Geometry check sheet. Reference: the model listing, model coordinates, mm. A direction names the side the tool comes from. Round coordinates to 2 decimals unless told otherwise and drop trailing zeros. Write each loop counter-clockwise with the first axis right and the second up, starting at its lowest first coordinate (ties: lowest second). Pieces come first, ordered by that corner, then holes. Notation, with made-up numbers: (-33, 6) -> (9, 6) arc R21 cw to (9, 23) -> close; hole circle Ø11 at (75, -39). An arc over 180 degrees is marked (long way). Use a Markdown table: item, result.
```python
from build123d import *

# Parameters (mm, degrees)
SKETCH2_R                        = 31.5
BOSS_EXTRUDE1_DEPTH              = 12
CBORE_FOR_M6_SHCS1_D             = 6.6
CBORE_FOR_M6_SHCS1_CBORE_D       = 11
CBORE_FOR_M6_SHCS1_CBORE_DEPTH   = 6.5
SKETCH5_R                        = 3.15
CUT_EXTRUDE1_DEPTH               = 6.5
BOSS_EXTRUDE2_DEPTH              = 27
CBORE_FOR_M2_5_SHCS1_D           = 2.7
CBORE_FOR_M2_5_SHCS1_CBORE_D     = 5.5
CBORE_FOR_M2_5_SHCS1_CBORE_DEPTH = 2.5
SKETCH9_W                        = 14.384523908
SKETCH9_H                        = 27
SKETCH9_W_2                      = 10
SKETCH9_H_2                      = 6
SKETCH9_W_3                      = 11.37493753
CUT_EXTRUDE2_DEPTH               = 15


with BuildPart() as part:
    # Sketch2 → Boss-Extrude1 (new body)
    with BuildSketch(Plane.XY):
        Circle(SKETCH2_R)
    extrude(amount=BOSS_EXTRUDE1_DEPTH)

    # CBORE for M6 SHCS1 (through all)
    with Locations(Plane.XY.offset(12)):
        with Locations((0, 25), (0, -25)):
            CounterBoreHole(CBORE_FOR_M6_SHCS1_D / 2, CBORE_FOR_M6_SHCS1_CBORE_D / 2, CBORE_FOR_M6_SHCS1_CBORE_DEPTH)

    # Sketch5 → Cut-Extrude1 (cut)
    with BuildSketch(Plane(origin=(0, 0, 0), x_dir=(-1, 0, 0), z_dir=(0, 0, -1))):
        with Locations((17.67766953, 17.67766953)):
            Circle(SKETCH5_R)
    extrude(amount=-CUT_EXTRUDE1_DEPTH, mode=Mode.SUBTRACT)

    # Sketch6 → Boss-Extrude2 (add)
    with BuildSketch(Plane(origin=(0, 0, 12), x_dir=(-1, 0, 0), z_dir=(0, 0, -1))):
        with BuildLine():
            Line((-31.379730719, -2.75), (31.379730719, -2.75))
            ThreePointArc((31.379730719, -2.75), (29.665019709, -10.594177913), (26.022826518, -17.75))
            Line((26.022826518, -17.75), (-26.022826518, -17.75))
            ThreePointArc((-26.022826518, -17.75), (-29.665019709, -10.594177913), (-31.379730719, -2.75))
        make_face()
    extrude(amount=-BOSS_EXTRUDE2_DEPTH)

    # CBORE for M2.5 SHCS1 (through all)
    with Locations(Plane(origin=(0, -2.75, 0), x_dir=(1, 0, 0), z_dir=(0, 1, 0))):
        with Locations((-9.995206811, -25), (14.004793189, -37), (-9.995206811, -37), (14.004793189, -25)):
            CounterBoreHole(CBORE_FOR_M2_5_SHCS1_D / 2, CBORE_FOR_M2_5_SHCS1_CBORE_D / 2, CBORE_FOR_M2_5_SHCS1_CBORE_DEPTH)

    # Sketch9 → Cut-Extrude2 (cut)
    with BuildSketch(Plane(origin=(0, -2.75, 0), x_dir=(1, 0, 0), z_dir=(0, 1, 0))):
        with Locations((-24.187468765, -25.5)):
            Rectangle(SKETCH9_W, SKETCH9_H)
        with Locations((6.504793189, -36)):
            Rectangle(SKETCH9_W_2, SKETCH9_H_2)
        with Locations((25.692261954, -36)):
            Rectangle(SKETCH9_W_3, SKETCH9_H_2)
    extrude(amount=-CUT_EXTRUDE2_DEPTH, mode=Mode.SUBTRACT)


solid = part.part
```
(1) Section check D-D on y = -16. Record the cut outline in (x, z), plus the area to 3 significant figures.
A:
| item | result |
|---|---|
| outline | (-27.13, 0) -> (27.13, 0) -> (27.13, 33) -> (20, 33) -> (20, 39) -> (11.5, 39) -> (11.5, 33) -> (1.5, 33) -> (1.5, 39) -> (-17, 39) -> (-17, 12) -> (-27.13, 12) -> close; hole circle Ø2.7 at (-10, 25); hole circle Ø2.7 at (-10, 37); hole circle Ø2.7 at (14, 25); hole circle Ø2.7 at (14, 37) |
| area | 1,720 mm2 |
(2) Access from +Z, -Z, +X, -X, +Y, -Y to the whole of each face (thin tool, end or side, straight path). Record for faces 1 (the face through (-9.9, -3.98, 34.25)), 2 (the face through (0, 21, 5.5)), 3 (the face through (-18, 18, 6.5)).
A:
| item | result |
|---|---|
| face 1 | +Y |
| face 2 | +Z |
| face 3 | -Z |
(3) Section check C-C on y = -25. Record the cut outline in (x, z).
A:
| item | result |
|---|---|
| outline | (-19.16, 0) -> (-3.3, 0) -> (-3.3, 5.5) -> (-5.5, 5.5) -> (-5.5, 12) -> (-19.16, 12) -> close; (3.3, 0) -> (19.16, 0) -> (19.16, 12) -> (5.5, 12) -> (5.5, 5.5) -> (3.3, 5.5) -> close |
(4) Release check for a two-part mould opening along X. For faces 4 (the face through (20.005, -10, 36)), 5 (the face through (16, -10, 39)), 6 (the face through (-10.353, -3.982, 22.273)) record: +X half, -X half, draft (parallel to the pull), parting line (faces both ways), or undercut.
A:
| item | result |
|---|---|
| face 4 | +X half |
| face 5 | draft |
| face 6 | undercut |
(5) Section check B-B on z = 25. Record the cut outline in (x, y), plus the area to 3 significant figures.
A:
| item | result |
|---|---|
| outline | (-17, -17.75) -> (-11.35, -17.75) -> (-11.35, -5.25) -> (-12.75, -5.25) -> (-12.75, -2.75) -> (-17, -2.75) -> close; (-8.65, -17.75) -> (12.65, -17.75) -> (12.65, -5.25) -> (11.25, -5.25) -> (11.25, -2.75) -> (-7.25, -2.75) -> (-7.25, -5.25) -> (-8.65, -5.25) -> close; (15.35, -17.75) -> (26.02, -17.75) arc R31.5 ccw to (31.38, -2.75) -> (16.75, -2.75) -> (16.75, -5.25) -> (15.35, -5.25) -> close |
| area | 601 mm2 |
(6) Thickness scan on line 1 (X direction, y = -4.1, z = 37); line 2 (Y direction, x = 0, z = 9); line 3 (X direction, y = -8.5, z = 37). Record the ranges inside material, lowest first.
A:
| item | result |
|---|---|
| line 1 | x = -17 to -12.75, -7.25 to 1.5, 16.75 to 20 |
| line 2 | y = -31.5 to -30.5, -19.5 to 19.5, 30.5 to 31.5 |
| line 3 | x = -17 to -11.35, -8.65 to 1.5, 11.5 to 12.65, 15.35 to 20 |
(7) Section check A-A on z = 37. Record the cut outline in (x, y), plus the area to 3 significant figures.
A:
| item | result |
|---|---|
| outline | (-17, -17.75) -> (-11.35, -17.75) -> (-11.35, -5.25) -> (-12.75, -5.25) -> (-12.75, -2.75) -> (-17, -2.75) -> close; (-8.65, -17.75) -> (1.5, -17.75) -> (1.5, -2.75) -> (-7.25, -2.75) -> (-7.25, -5.25) -> (-8.65, -5.25) -> close; (11.5, -17.75) -> (12.65, -17.75) -> (12.65, -5.25) -> (11.5, -5.25) -> close; (15.35, -17.75) -> (20, -17.75) -> (20, -2.75) -> (16.75, -2.75) -> (16.75, -5.25) -> (15.35, -5.25) -> close |
| area | 311 mm2 |
(8) Gauge pin test, flat ends, axial feed: pin 1 Ø4.5 at (x, z) = (-10, 25) entering from +Y; pin 2 Ø7 at (x, z) = (-10, 37) entering from +Y; pin 3 Ø6.5 at (y, z) = (-9, 37) entering from +X; pin 4 Ø5.5 at (x, y) = (0, -25) entering from -Z. Record the tip position at first contact, or that the pin passes through.
A:
| item | result |
|---|---|
| pin 1 | stops at y = -5.25 |
| pin 2 | stops at y = -2.75 |
| pin 3 | stops at x = 20 |
| pin 4 | passes through |
